Part model, mm, in its own coordinate system. A direction names the side the tool comes from. Give positions to 0.01 mm unless a question says otherwise; leave off trailing zeros. Loops run counter-clockwise (first coordinate to the right, second up) from the corner with the lowest first, then second, coordinate; pieces in that order, holes last. Notation, with made-up numbers: M -15,81.25 L 10,81.25 A21 ccw 10,91.25 Z; hole C -11,67 d4. An arc over 180 degrees is marked long. Put each result on its own line as item: value. Start each with the question number.
Autodesk Inventor part; units mm, degrees
ref_plane "YZ Plane" through (0, 0, 0) normal (1, 0, 0) x (0, 1, 0)
ref_plane "XZ Plane" through (0, 0, 0) normal (0, 1, 0) x (-1, 0, 0)
ref_plane "XY Plane" through (0, 0, 0) normal (0, 0, 1) x (1, 0, 0)
sketch "Sketch1" plane through (0, 0, 0) normal (0, 0, 1) x (1, 0, 0)
  line L0 (0, 0) -> (0, 40)
  line L1 (0, 0) -> (63, 0)
  line L2 (63, 0) -> (63, 5)
  line L3 (63, 5) -> (9, 5)
  arc A0 (9, 40) -> (0, 40) centre (4.5, 40) ccw
  line L4 (9, 40) -> (9, 5)
  circle A1 centre (4.5, 40) radius 2.5
  dimension "d0" = 40
  dimension "d2" = 5
  dimension "d6" = 4.5
  dimension "d7" = 5
  dimension "d8" = 9
  dimension "d9" = 54
  dimension "d47" = 32.5
extrude "Extrusion1" add sketch "Sketch1" along normal blind 20
sketch "Sketch2" plane through (9, 5, 0) normal (0, 1, 0) x (1, 0, 0)
  line L0 (0, 0) -> (0, -20)
  circle A0 centre (26, -10) radius 10
  line L1 (0, 0) -> (54, 0)
  circle A1 centre (52, -10) radius 2
  line L2 (54, 0) -> (54, -20)
  point P0 (-9, 0)
  dimension "d14" = 20
  dimension "d16" = 26
  dimension "d20" = 4
  dimension "d21" = 10
  dimension "d22" = 14
sketch "Sketch6" plane through (9, 5, 0) normal (1, 0, 0) x (0, 0, -1)
  point P0 (0, -5)
sketch "Sketch7" plane through (9, 5, 0) normal (1, 0, 0) x (0, 0, -1)
  line L0 (-10, 41.0364) -> (-10, 39.6436)
  line L1 (0, 39.5) -> (-20, 39.5)
  line L2 (-2.5, 39.5) -> (-2.5, 25.5)
  line L3 (-17.5, 39.5) -> (-17.5, 25.5)
  line L4 (-17.5, 39.5) -> (-2.5, 39.5)
  line L5 (0, 32.5) -> (-20, 32.5)
  line L6 (-17.5, 25.5) -> (-2.5, 25.5)
  point P0 (0, -5)
  dimension "d40" = 14
  dimension "d41" = 14
  dimension "d42" = 15
extrude "Extrusion5" cut sketch "Sketch7" against normal blind 14
sketch "Sketch8" plane through (0, 0, 0) normal (0, 0, -1) x (-1, 0, 0)
  point P0 (0, 0)
extrude "Extrusion6" add sketch "Sketch2" along normal blind 20
sketch "Sketch9" plane through (35, 25, 10) normal (0, 1, 0) x (1, 0, 0)
  circle A0 centre (0, 0) radius 9
  point P0 (-35, 10)
  dimension "d50" = 18
extrude "Extrusion7" cut sketch "Sketch9" against normal blind 25
sketch "Sketch10" plane through (9, 5, 20) normal (0, 1, 0) x (1, 0, 0)
  line L0 (3, 8) -> (7, 8)
  line L1 (7, 8) -> (7, 12)
  line L2 (7, 12) -> (3, 12)
  line L3 (3, 12) -> (3, 8)
  line L4 (26, 0) -> (0, 0)
  line L5 (0, 2.5) -> (0, 17.5)
  point P0 (-9, 20)
  dimension "d53" = 4
  dimension "d54" = 4
  dimension "d55" = 8
  dimension "d56" = 3
extrude "Extrusion8" add sketch "Sketch10" along normal blind 6
sketch "Sketch11" plane through (16, 5, 8) normal (0, 0, -1) x (-1, 0, 0)
  line L0 (1, 3.8) -> (2, 3.8)
  line L1 (1, 3.8) -> (0, 2.8)
  line L2 (4, 0) -> (4, 6)
  line L3 (7, 0) -> (-19, 0)
  line L4 (0, 0) -> (4, 0)
  line L5 (0, 2.8) -> (0, 0)
  line L6 (0, 0) -> (2, 3.8)
  point P0 (16, -5)
  dimension "d59" = 2
  dimension "d60" = 1
  dimension "d61" = 3.8
  dimension "d62" = 2.8
extrude "Extrusion9" cut sketch "Sketch11" against normal blind 4
equation "\"d21\" = d19"
equation "\"d40\" = d41"
equation "\"d19\" = 0.5 * d14"
properties part number "ValveBaseMk2.2"
1) Band-saw the part on D-D on x = 61. Give the cut face in (y, z).
2) Which spindle directions (+Z, -Z, +X, -X, +Y, -Y) get a long thin tool onto all of the face, cutting with end or side? Do faces 4 (the flat face through (61, 25, 10)), 5 (the flat face through (14, 8, 12)), 6 (the flat face through (14, 8, 8)), 7 (the cylindrical face through (32.83, 14.86, 0.24)). Say none if no direction does.
3) Mould opens along X. For faces 1 (the cylindrical face through (4.4, 44.5, 18.7)), 2 (the flat face through (5, 36, 17.5)), 3 (the flat face through (15, 6.9, 10)) say: +X half, -X half, draft (parallel to the pull), parting line (faces both ways), or undercut.
4) Band-saw the part on C-C on y = 33.5. Give the cut face in (x, z).
5) Band-saw the part on A-A on y = 22. Give the cut face in (x, z).
6) Pin check, flat tips, straight feed: pin 1 Ø2.5 at (y, z) = (9.5, 9.5) entering from +X; pin 2 Ø3 at (x, z) = (60, 11) entering from +Y; pin 3 Ø4 at (y, z) = (26, 16) entering from +X; pin 4 Ø3 at (x, z) = (15, 10) entering from +Y. Stop position of each tip, or through.
7) Wall check: L1, parallel to X at y = 13, z = 10; L2, parallel to Z at x = 35, y = 19.25; L3, parallel to X at y = 40, z = 18.1. Give the ranges that are in metal, low to high.
8) Band-saw the part on B-B on x = 4.5. Give the cut face in (y, z).
Evaluation:
1. outline: M 0,0 L 5,0 L 5,8 L 25,8 L 25,12 L 5,12 L 5,20 L 0,20 Z
2. face 4: +Z, -Z, +X, +Y
2. face 5: +Z, +Y
2. face 6: -Z, +Y
2. face 7: +Y
3. face 1: parting line
3. face 2: draft
3. face 3: undercut
4. outline: M 0,0 L 9,0 L 9,2.5 L 0,2.5 Z; M 0,17.5 L 9,17.5 L 9,20 L 0,20 Z
5. outline: M 0,0 L 9,0 L 9,20 L 0,20 Z; C 35,10 d20; C 61,10 d4; hole C 35,10 d18
6. pin 1: x = 63
6. pin 2: y = 25
6. pin 3: x = 44.04
6. pin 4: y = 11
7. L1: 0 to 9, 25 to 26, 44 to 45, 59 to 63
7. L2: 0 to 1, 19 to 20
7. L3: 0 to 2, 7 to 9
8. outline: M 0,0 L 37.5,0 L 37.5,2.5 L 30.5,2.5 L 30.5,17.5 L 37.5,17.5 L 37.5,20 L 0,20 Z; M 42.5,0 L 44.5,0 L 44.5,2.5 L 42.5,2.5 Z; M 42.5,17.5 L 44.5,17.5 L 44.5,20 L 42.5,20 Z
